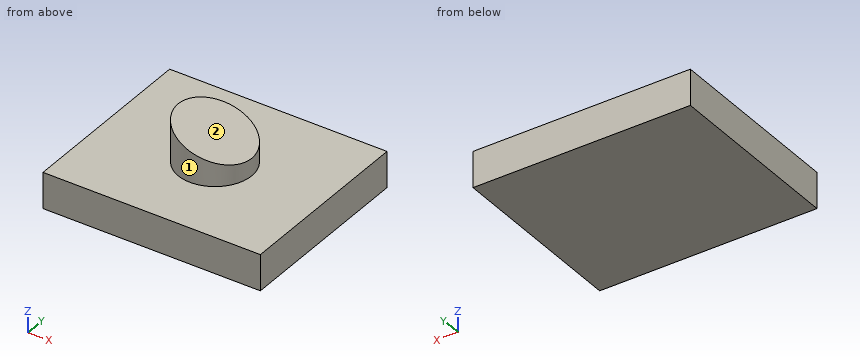
from build123d import *

# Parameters (mm, degrees)
F0_W     = 108.90334
F0_H     = 93.113952
F1_DEPTH = 18.034
F2_R     = 18.445574
F3_DEPTH = 54.61
F5_DEPTH = 25.4


with BuildPart() as f1:
    # F0 (on Top) → F1 (new body)
    with BuildSketch(Plane.XY):
        Rectangle(F0_W, F0_H)
    extrude(amount=-F1_DEPTH)

    # F2 (on Top) → F3 (join)
    with BuildSketch(Plane.XY):
        Circle(F2_R)
    extrude(amount=F3_DEPTH)

    # F4 (on Front) → F5 (cut, symmetric)
    with BuildSketch(Plane.XZ):
        Polygon((-27.631808, 92.519648), (-27.631808, 25.349762), (42.751096, 0), (42.751096, 25.349762), (42.751096, 92.519648), align=None)
    extrude(amount=F5_DEPTH, both=True, mode=Mode.SUBTRACT)


solid = f1.part
Read the model definition and answer for the solid it produces. Units are mm, in the model's axes. Face numbers are marked on the shaded views. A direction names the side the tool comes from. Give positions to 0.01 mm unless a question says otherwise; leave off trailing zeros. Write each loop counter-clockwise with the first axis right and the second up, starting at its lowest first coordinate (ties: lowest second). Pieces come first, ordered by that corner, then holes. Notation, with made-up numbers: (23, 84) - (62, 84) arc R27 ccw to (62, 119) - close; hole circle Ø10 at (-13.5, 43.25). An arc over 180 degrees is marked (long way). Answer in a Markdown table with one row per item. Add a question column.
Item 1: Section C-C, the plane z = 18 is taken. Write down the section's boundary in (x, y), and give its area (3 significant figures).
Item 2: Find the intervals of material crossed by L1, parallel to Z at x = 22.5, y = -2; L2, parallel to X at y = 14, z = 6.5; L3, parallel to X at y = -4, z = 3.5, in increasing order.
Item 3: A tool of negligible diameter and unlimited length cuts with its end or side. For the marked faces 1 and 2, from which of +Z, -Z, +X, -X, +Y, -Y can it reach the whole face along a straight path? Write none if from no direction.
Item 4: Section A-A, the plane y = 0 is taken. Write down the section's boundary in (x, z), and give its area (3 significant figures).
Item 5: Section D-D, the plane y = -22.5 is taken. Write down the section's boundary in (x, z), and give its area (3 significant figures).
Item 6: Section B-B, the plane x = 0 is taken. Write down the section's boundary in (y, z).
Item 7: Flat-ended cylindrical pins translate along their axes: P1, Ø12, axis at y = 3, z = 5.5, coming from the -X side; P2, Ø1, axis at x = -8, z = 7, coming from the -Y side. Find the tip coordinate at first contact, or state that the pin passes through.
Recorded:
| question | item | result |
|---|---|---|
| 1 | outline | (-7.23, -16.97) - (-7.23, 16.97) arc R18.45 ccw to start |
| 1 | area | 275 mm2 |
| 2 | L1 | z = -18.03 to 0 |
| 2 | L2 | x = -12.01 to 12.01 |
| 2 | L3 | x = -18.01 to 18.01 |
| 3 | face 1 | +Z |
| 3 | face 2 | +Z, +X, +Y, -Y |
| 4 | outline | (-54.45, -18.03) - (54.45, -18.03) - (54.45, 0) - (18.45, 0) - (18.45, 8.75) - (-18.45, 22.04) - (-18.45, 0) - (-54.45, 0) - close |
| 4 | area | 2,530 mm2 |
| 5 | outline | (-54.45, -18.03) - (54.45, -18.03) - (54.45, 0) - (-54.45, 0) - close |
| 5 | area | 1,960 mm2 |
| 6 | outline | (-46.56, -18.03) - (46.56, -18.03) - (46.56, 0) - (18.45, 0) - (18.45, 15.4) - (-18.45, 15.4) - (-18.45, 0) - (-46.56, 0) - close |
| 7 | P1 | stops at x = -54.45 |
| 7 | P2 | stops at y = -16.85 |
